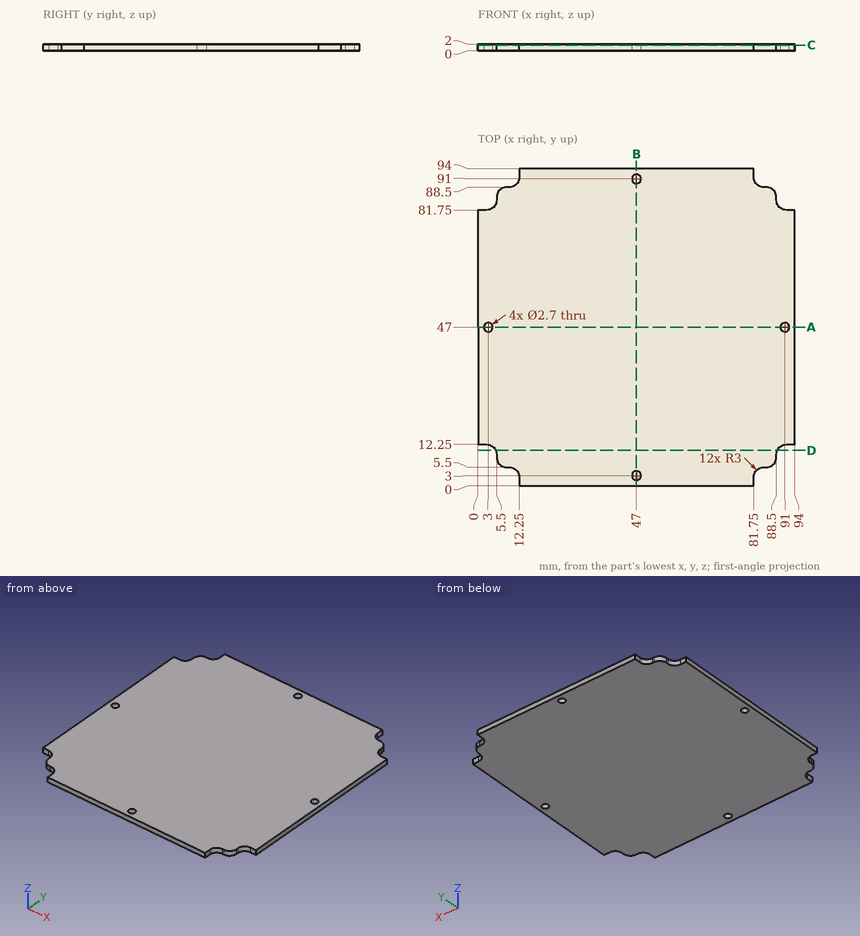
Drawing for the job (mm, zero at the part's lowest x, y, z). Give positions to 0.01 mm unless a question says otherwise; leave off trailing zeros. Order: outer loops, then holes, each group sorted by start corner. A loop starts at its lowest first (then second) coordinate and runs counter-clockwise, first axis right, second up. Notation, with made-up numbers: M 23,-37.5 L 76,-37.5 A21 cw 76,-20.5 Z; hole C 35.25,63 d3. An arc over 180 degrees is marked long. Use a Markdown table: item, result. Add a question column.
(1) Drop flat-ended pins along their axis: P1, Ø2, axis at x = 47, y = 91, coming from the +Z side; P2, Ø0.6, axis at x = 93, z = 0.5, coming from the -Y side; P3, Ø0.6, axis at y = 9, z = 1, coming from the +X side; P4, Ø1, axis at y = 1, z = 1, coming from the +X side. Give the stop position or say it passes through.
(2) Saw through at C-C, the plane z = 1.7. Give the number of separate pieces and of enclosed holes in the cut face, and give its area (3 significant figures).
(3) Probe line 1 along Y through (x, z) = (47, 0.9); line 2 along Y through (x, z) = (48, 0.75); line 3 along Y through (x, z) = (4, 1.9). List the from-to ranges inside material, lowest first. Write a range as [from, to].
(4) Saw through at D-D, the plane y = 10.5. Give the cut face in (x, z).
(5) Saw through at A-A, the plane y = 47. Give the cut face in (x, z).
Answer key:
| question | item | result |
|---|---|---|
| 1 | P1 | through |
| 1 | P2 | y = 12.25 |
| 1 | P3 | x = 88.5 |
| 1 | P4 | x = 81.75 |
| 2 | separate pieces | 1 |
| 2 | enclosed holes | 4 |
| 2 | area | 8,400 mm^2 |
| 3 | line 1 | [0, 1.65], [4.35, 89.65], [92.35, 94] |
| 3 | line 2 | [0, 2.09], [3.91, 90.09], [91.91, 94] |
| 3 | line 3 | [11.85, 46.09], [47.91, 82.15] |
| 4 | outline | M 5.23,0 L 88.77,0 L 88.77,2 L 5.23,2 Z |
| 5 | outline | M 0,0 L 1.65,0 L 1.65,2 L 0,2 Z; M 4.35,0 L 89.65,0 L 89.65,2 L 4.35,2 Z; M 92.35,0 L 94,0 L 94,2 L 92.35,2 Z |
